```python
from build123d import *

# Parameters (mm, degrees)
BOSS_EXTRUDE1_DEPTH = 23.8125
SKETCH2_R           = 7.9121
CUT_EXTRUDE1_DEPTH  = 16.875
FILLET1_R           = 0.79375


with BuildPart() as part:
    # Sketch1 → Boss-Extrude1 (new body, symmetric)
    with BuildSketch(Plane.XY):
        Polygon((15.478125, 15.875), (-15.478125, 15.875), (-15.478125, 11.1125), (-23.8125, 11.1125), (-23.8125, 0), (23.8125, 0), (23.8125, 11.1125), (15.478125, 11.1125), align=None)
    extrude(amount=BOSS_EXTRUDE1_DEPTH, both=True)

    # Sketch2 → Cut-Extrude1 (cut, through all)
    with BuildSketch(Plane(origin=(0, 15.875, 0), x_dir=(1, 0, 0), z_dir=(0, 1, 0))):
        Circle(SKETCH2_R)
    extrude(amount=-CUT_EXTRUDE1_DEPTH, mode=Mode.SUBTRACT)

    # Fillet1
    fillet1_edges = [part.edges().sort_by_distance(p)[0] for p in [
        (-23.8125, 0, 0),
        (-15.478125, 15.875, 0),
        (15.478125, 15.875, 0),
        (23.8125, 0, 0),
    ]]
    fillet(fillet1_edges, radius=FILLET1_R)


solid = part.part
```
Geometry check sheet. Reference: the model listing, model coordinates, mm. A direction names the side the tool comes from. Coordinates: 2 decimals unless noted, no trailing zeros. Order: outer loops, then holes, each group sorted by start corner. A loop starts at its lowest first (then second) coordinate and runs counter-clockwise, first axis right, second up.
Item 1: Tool access check on faces 4 (the flat face through (15.478, 13, 0)), 5 (the flat face through (-20, 11.112, 0)), 6 (the flat face through (-11, 0, 0)). Record the directions out of +Z, -Z, +X, -X, +Y, -Y that give a thin tool (end or side, any length) a straight path to the whole face; none if there is none.
Item 2: Section check C-C (y = 2.75). Enter the section's corners in (x, z).
Item 3: Scan lines: line 1 along Z through (x, y) = (0, 11.25); line 2 along X through (y, z) = (12, 0). Record each from-to range of solid material in increasing order.
Item 4: Depth check by flat-ended pin: pin 1 (4 mm diameter, centred on y = 13, z = -13, fed in from -X); pin 2 (4 mm diameter, centred on x = -20, z = 1, fed in from +Y). Enter the tip coordinate at first touch or a pass-through.
Item 5: Mould release check, pull along Z, two halves, no side actions. Record for faces 1 (the flat face through (23.812, 6, 0)), 2 (the flat face through (0, 6, 23.812)), 3 (the cylindrical face through (-1.715, 8.049, 7.724)): released by +Z, released by -Z, zero draft, split by the parting line, or undercut.
Item 6: Section check D-D (z = -15). Enter the section's corners in (x, y) (1 decimal), plus the area to 3 significant figures.
Item 7: Section check A-A (z = 0). Enter the section's corners in (x, y) (1 decimal).
Item 8: Section check B-B (x = 0). Enter the section's corners in (y, z) (1 decimal).
Check sheet entries:
1. face 4: +Z, -Z, +X, +Y
1. face 5: +Z, -Z, -X, +Y
1. face 6: +Z, -Z, +X, -X, -Y
2. outline: (-23.81, -23.81) - (23.81, -23.81) - (23.81, 23.81) - (-23.81, 23.81) - close; hole circle Ø15.82 at (0, 0)
3. line 1: z = -23.81 to -7.91, 7.91 to 23.81
3. line 2: x = -15.48 to -7.91, 7.91 to 15.48
4. pin 1: stops at x = -23.81
4. pin 2: stops at y = 11.11
5. face 1: zero draft
5. face 2: released by +Z
5. face 3: undercut
6. outline: (-23.8, 0.8) arc R0.8 ccw to (-23, 0) - (23, 0) arc R0.8 ccw to (23.8, 0.8) - (23.8, 11.1) - (15.5, 11.1) - (15.5, 15.1) arc R0.8 ccw to (14.7, 15.9) - (-14.7, 15.9) arc R0.8 ccw to (-15.5, 15.1) - (-15.5, 11.1) - (-23.8, 11.1) - close
6. area: 676 mm2
7. outline: (-23.8, 0.8) arc R0.8 ccw to (-23, 0) - (-7.9, 0) - (-7.9, 15.9) - (-14.7, 15.9) arc R0.8 ccw to (-15.5, 15.1) - (-15.5, 11.1) - (-23.8, 11.1) - close; (7.9, 0) - (23, 0) arc R0.8 ccw to (23.8, 0.8) - (23.8, 11.1) - (15.5, 11.1) - (15.5, 15.1) arc R0.8 ccw to (14.7, 15.9) - (7.9, 15.9) - close
8. outline: (0, -23.8) - (15.9, -23.8) - (15.9, -7.9) - (0, -7.9) - close; (0, 7.9) - (15.9, 7.9) - (15.9, 23.8) - (0, 23.8) - close
